The drawing under review shows one solid part. Ordinate dimensions are in mm from its lowest x, y, z. Round coordinates to 2 decimals unless told otherwise and drop trailing zeros. Write each loop counter-clockwise with the first axis right and the second up, starting at its lowest first coordinate (ties: lowest second). Pieces come first, ordered by that corner, then holes.
Item 1: Add section B-B (y = 1). Give the boundary of the cut face in (x, z).
Item 2: To check wall thickness, follow L1, parallel to Z at x = 2.5, y = 1.2; L2, parallel to Z at x = 3.5, y = 2.4; L3, parallel to X at y = 2.2, z = 3.5. State the ranges of each line that lie inside material, in increasing order.
Item 3: Add section C-C (x = 4.1). Give the boundary of the cut face in (y, z), plus the area to 3 significant figures.
Item 4: Clearance check with a flat-ended pin moving along its axis: pin 1 Ø2 at (x, z) = (2.5, 32.5) entering from -Y. State where the tip first meets the part, or that it passes through.
Item 5: Add section A-A (x = 2.5). Give the boundary of the cut face in (y, z).
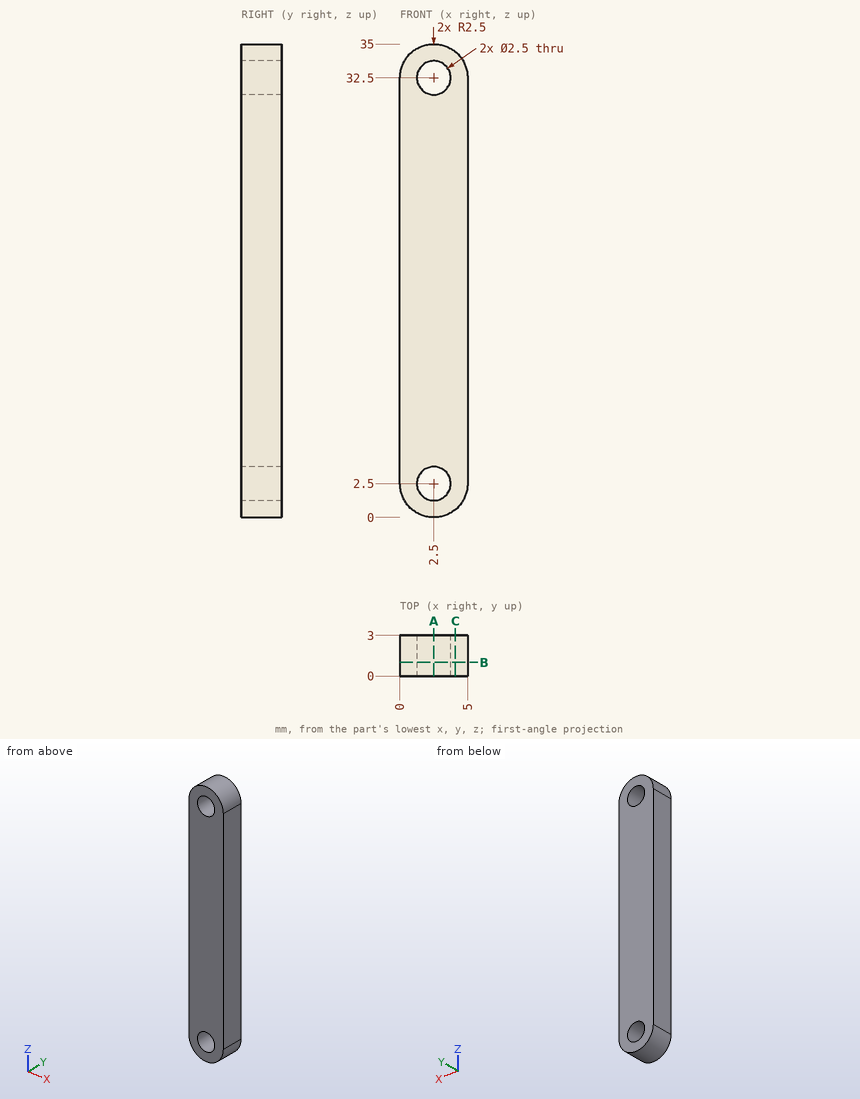
Numbers:
1. outline: (0, 2.5) arc R2.5 ccw to (5, 2.5) - (5, 32.5) arc R2.5 ccw to (0, 32.5) - close; hole circle Ø2.5 at (2.5, 2.5); hole circle Ø2.5 at (2.5, 32.5)
2. L1: z = 0 to 1.25, 3.75 to 31.25, 33.75 to 35
2. L2: z = 0.21 to 1.75, 3.25 to 31.75, 33.25 to 34.79
2. L3: x = 0 to 1.75, 3.25 to 5
3. outline: (0, 0.58) - (3, 0.58) - (3, 34.42) - (0, 34.42) - close
3. area: 102 mm2
4. pin 1: passes through
5. outline: (0, 0) - (3, 0) - (3, 1.25) - (0, 1.25) - close; (0, 3.75) - (3, 3.75) - (3, 31.25) - (0, 31.25) - close; (0, 33.75) - (3, 33.75) - (3, 35) - (0, 35) - close
